```python
from build123d import *


with BuildPart() as f3:
    # F0 (on Top) → F3 section 0
    with BuildSketch(Plane.XY, mode=Mode.PRIVATE) as f3_s0:
        Polygon((50.418489, 87.327384), (0, 100.836977), (-50.418489, 87.327384), (-87.327384, 50.418489), (-100.836977, 0), (-87.327384, -50.418489), (-50.418489, -87.327384), (0, -100.836977), (50.418489, -87.327384), (87.327384, -50.418489), (100.836977, 0), (87.327384, 50.418489), align=None)
    loft([f3_s0.sketch, Vertex(0, 0, 254)])


solid = f3.part
```
Can you work these out from the model? Positions are in its coordinate system, mm. Round coordinates to 2 decimals unless told otherwise and drop trailing zeros. Loops run counter-clockwise (first coordinate to the right, second up) from the corner with the lowest first, then second, coordinate; pieces in that order, holes last. Notation, with made-up numbers: (86.25, 1) -> (112.25, 1) arc R20 cw to (112.25, 24) -> close; hole circle Ø8 at (46.25, -21). An arc over 180 degrees is marked (long way). Answer in a Markdown table with one row per item.
Item 1: Will these pins go through, and if not, where does the flat tip stop? P1, Ø3, axis at x = -15, z = 141.5, coming from the -Y side; P2, Ø4, axis at x = -6, z = 223.5, coming from the +Y side; P3, Ø4, axis at y = -23, z = 133, coming from the +X side.
Answer block:
| item | result |
|---|---|
| P1 | y = -41.36 |
| P2 | y = 11.46 |
| P3 | x = 42.83 |
Item 2: If I drill on probe 1 along X at (y, z) = (-63, 38.5); probe 2 along Y at (x, z) = (62, 57); probe 3 along Y at (x, z) = (20.5, 157), over which ranges is the centre line in solid material (lowest first)?
Answer block:
| item | result |
|---|---|
| probe 1 | -53.87 to 53.87 |
| probe 2 | -44.83 to 44.83 |
| probe 3 | -32.1 to 32.1 |
Item 3: Suppose I cut it at B-B, the plane y = -4.5. List the corners of the cut face in (x, z) for me.
Answer block:
| item | result |
|---|---|
| outline | (-99.63, 0) -> (99.63, 0) -> (7.79, 231.33) -> (2.6, 240.91) -> (0, 242.66) -> (-2.6, 240.91) -> (-7.79, 231.33) -> close |
Item 4: Suppose I cut it at D-D, the plane z = 71. List the corners of the cut face in (x, y) for me.
Answer block:
| item | result |
|---|---|
| outline | (-72.65, 0) -> (-62.92, -36.33) -> (-36.33, -62.92) -> (0, -72.65) -> (36.33, -62.92) -> (62.92, -36.33) -> (72.65, 0) -> (62.92, 36.33) -> (36.33, 62.92) -> (0, 72.65) -> (-36.33, 62.92) -> (-62.92, 36.33) -> close |
Item 5: Suppose I cut it at C-C, the plane x = 9. List the corners of the cut face in (y, z) for me, plus the area to 3 significant figures.
Answer block:
| item | result |
|---|---|
| outline | (-98.43, 0) -> (98.43, 0) -> (15.59, 208.66) -> (5.2, 227.82) -> (0, 231.33) -> (-5.2, 227.82) -> (-15.59, 208.66) -> close |
| area | 24,200 mm² |
Item 6: Suppose I cut it at A-A, the plane z = 146. List the corners of the cut face in (x, y) for me, plus the area to 3 significant figures.
Answer block:
| item | result |
|---|---|
| outline | (-42.88, 0) -> (-37.13, -21.44) -> (-21.44, -37.13) -> (0, -42.88) -> (21.44, -37.13) -> (37.13, -21.44) -> (42.88, 0) -> (37.13, 21.44) -> (21.44, 37.13) -> (0, 42.88) -> (-21.44, 37.13) -> (-37.13, 21.44) -> close |
| area | 5,510 mm² |
